Here's how the part is built. I have some questions about the finished solid (model axes, mm). Face numbers are marked on the shaded views. A direction names the side the tool comes from. Give positions to 0.01 mm unless a question says otherwise; leave off trailing zeros. Write each loop counter-clockwise with the first axis right and the second up, starting at its lowest first coordinate (ties: lowest second). Pieces come first, ordered by that corner, then holes. Notation, with made-up numbers: (-27.75, -14) -> (-3.75, -14) arc R19 ccw to (-3.75, 18) -> close; hole circle Ø2 at (8, 40). An arc over 180 degrees is marked (long way). Return JSON: item names as keys, results as strings.
from build123d import *

# Parameters (mm, degrees)
SKETCH1_W           = 47
SKETCH1_H           = 33
BOSS_EXTRUDE1_DEPTH = 34
SKETCH2_W           = 33
SKETCH2_H           = 8
CUT_EXTRUDE1_DEPTH  = 22
SKETCH3_W           = 12
SKETCH3_H           = 15
CUT_EXTRUDE2_DEPTH  = 17


with BuildPart() as part:
    # Sketch1 → Boss-Extrude1 (new body)
    with BuildSketch(Plane.XY):
        with Locations((2.68144213, 1.197180866)):
            Rectangle(SKETCH1_W, SKETCH1_H)
    extrude(amount=BOSS_EXTRUDE1_DEPTH)

    # Sketch2 → Cut-Extrude1 (cut)
    with BuildSketch(Plane.XY.offset(34)):
        with Locations((9.68144213, 13.697180866)):
            Rectangle(SKETCH2_W, SKETCH2_H)
    extrude(amount=-CUT_EXTRUDE1_DEPTH, mode=Mode.SUBTRACT)

    # Sketch3 → Cut-Extrude2 (cut)
    with BuildSketch(Plane(origin=(26.18144213, 0, 0), x_dir=(0, 0, -1), z_dir=(1, 0, 0))):
        with Locations((-28, -4.802819134)):
            Rectangle(SKETCH3_W, SKETCH3_H)
        Polygon((-12, 2.697180866), (-12, 9.697180866), (-34, 9.697180866), (-34, 2.697180866), (-22, 2.697180866), align=None)
    extrude(amount=-CUT_EXTRUDE2_DEPTH, mode=Mode.SUBTRACT)


solid = part.part
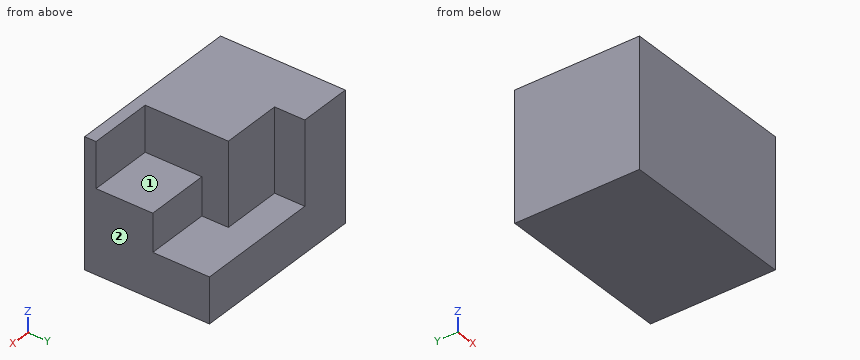
1. Which directions (+Z, -Z, +X, -X, +Y, -Y) give clear straight access to the entire face, cutting with the end or side of a thin tool? Please do the marked faces 1 and 2.
Taken from the geometry:
{"face 1": "+Z, +X, +Y", "face 2": "+Z, -Z, +X, +Y, -Y"}
2. Suppose I cut it at C-C, the plane y = -9.5. List the corners of the cut face in (x, z) for me, and give its area (3 significant figures).
Taken from the geometry:
{"outline": "(-20.82, 0) -> (26.18, 0) -> (26.18, 22) -> (9.18, 22) -> (9.18, 34) -> (-20.82, 34) -> close", "area": "1,390 mm²"}
3. Suppose I cut it at B-B, the plane z = 29.5. List the corners of the cut face in (x, y) for me, and give its area (3 significant figures).
Taken from the geometry:
{"outline": "(-20.82, -15.3) -> (26.18, -15.3) -> (26.18, -12.3) -> (9.18, -12.3) -> (9.18, 9.7) -> (-6.82, 9.7) -> (-6.82, 17.7) -> (-20.82, 17.7) -> close", "area": "913 mm²"}
4. For pin 1 Ø4.5 at (x, y) = (13.5, 7.5) entering from +Z; pin 2 Ø4 at (y, z) = (13.5, 17.5) entering from +X; pin 3 Ø17.5 at (x, z) = (2, 23) entering from +Y, each with a flat end and sliding along its axis, tell me the tip position at first contact or that it passes through.
Taken from the geometry:
{"pin 1": "stops at z = 12", "pin 2": "stops at x = -6.82", "pin 3": "stops at y = 9.7"}
5. Suppose I cut it at A-A, the plane x = 14. List the corners of the cut face in (y, z) for me.
Taken from the geometry:
{"outline": "(-15.3, 0) -> (17.7, 0) -> (17.7, 12) -> (2.7, 12) -> (2.7, 22) -> (-12.3, 22) -> (-12.3, 34) -> (-15.3, 34) -> close"}
6. If I drill on line 1 (Y direction, x = 7, z = 27); line 2 (X direction, y = 14, z = 27); line 3 (Z direction, x = 24.5, y = -10), over which ranges is the centre line in solid material (lowest first)? Write a range as [from, to].
Taken from the geometry:
{"line 1": "y = [-15.3, 9.7]", "line 2": "x = [-20.82, -6.82]", "line 3": "z = [0, 22]"}
7. Suppose I cut it at D-D, the plane y = 11.5. List the corners of the cut face in (x, z) for me, and give its area (3 significant figures).
Taken from the geometry:
{"outline": "(-20.82, 0) -> (26.18, 0) -> (26.18, 12) -> (-6.82, 12) -> (-6.82, 34) -> (-20.82, 34) -> close", "area": "872 mm²"}
